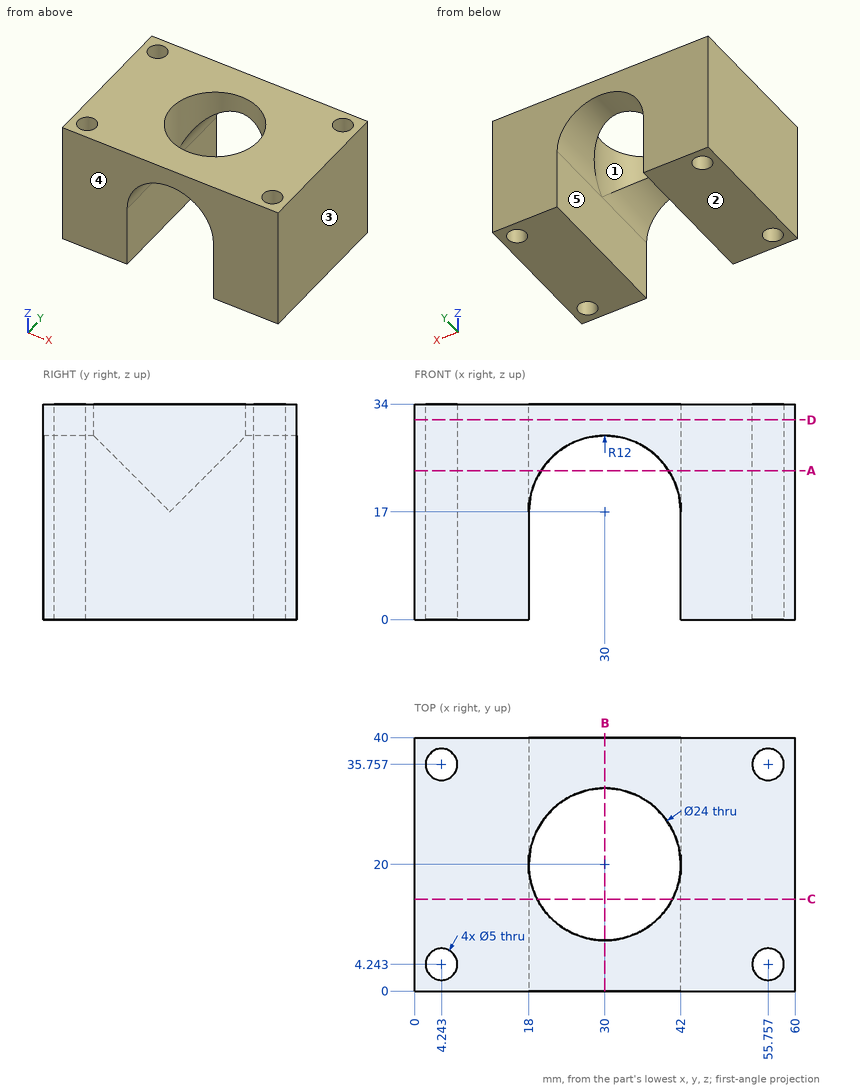
Design review of the part shown in the three views and the two pictorial views. Dimensions are in mm from the part's minimum x, y and z. A direction names the side the tool comes from. Round coordinates to 2 decimals unless told otherwise and drop trailing zeros. Loops run counter-clockwise (first coordinate to the right, second up) from the corner with the lowest first, then second, coordinate; pieces in that order, holes last. Notation, with made-up numbers: M 63,26 L 81,26 A18 ccw 81,35 Z; hole C 51,10.25 d10. An arc over 180 degrees is marked long. Answer as a JSON object with one key per item and string values.
Item 1: Clearance check with a flat-ended pin moving along its axis: P1, Ø8, axis at x = 24.5, y = 22.5, coming from the +Z side. State where the tip first meets the part, or that it passes through.
Answer sheet:
{"P1": "passes through"}
Item 2: We need section D-D on z = 31.5. Give the boundary of the cut face in (x, y), and give its area (3 significant figures).
Answer sheet:
{"outline": "M 0,0 L 60,0 L 60,40 L 0,40 Z; hole C 4.24,4.24 d5; hole C 4.24,35.76 d5; hole C 30,20 d24; hole C 55.76,4.24 d5; hole C 55.76,35.76 d5", "area": "1,870 mm^2"}
Item 3: We need section B-B on x = 30. Give the boundary of the cut face in (y, z), and give its area (3 significant figures).
Answer sheet:
{"outline": "M 0,29 L 8,29 L 8,34 L 0,34 Z; M 32,29 L 40,29 L 40,34 L 32,34 Z", "area": "80.0 mm^2"}
Item 4: We need section C-C on y = 14.5. Give the boundary of the cut face in (x, z) (1 decimal).
Answer sheet:
{"outline": "M 0,0 L 18,0 L 18,17 A12 cw 19.3,22.5 L 19.3,34 L 0,34 Z; M 40.7,22.5 A12 cw 42,17 L 42,0 L 60,0 L 60,34 L 40.7,34 Z"}
Item 5: Machinability: for the marked faces 4 and 5, which of the approach directions +Z, -Z, +X, -X, +Y, -Y give a long, thin tool a straight path to every point of the face, cutting with its end or side? Answer none if there is none.
Answer sheet:
{"face 4": "+Z, -Z, +X, -X, -Y", "face 5": "-Z, +Y, -Y"}
Item 6: We need section A-A on z = 23.5. Give the boundary of the cut face in (x, y), and give its area (3 significant figures).
Answer sheet:
{"outline": "M 0,0 L 19.91,0 L 19.91,13.5 A12 cw 19.91,26.5 L 19.91,40 L 0,40 Z; M 40.09,0 L 60,0 L 60,40 L 40.09,40 L 40.09,26.5 A12 cw 40.09,13.5 Z; hole C 4.24,4.24 d5; hole C 4.24,35.76 d5; hole C 55.76,4.24 d5; hole C 55.76,35.76 d5", "area": "1,480 mm^2"}
Item 7: Wall thickness on L1, parallel to Y at x = 4.5, z = 5.5; L2, parallel to X at y = 19.5, z = 26; L3, parallel to Y at x = 6.5, z = 27 (1 decimal): over which ranges is each line inside the solid? List them lowest first. Write a range as from..to.
Answer sheet:
{"L1": "y = 0..1.76, 6.73..33.27, 38.24..40", "L2": "x = 0..18.01, 41.99..60", "L3": "y = 0..3.2, 5.3..34.7, 36.8..40"}
Item 8: The part is to be moulded in two halves that separate along X. For the marked faces 1, 2 and 3, say which applies: pulls with the +X half, pulls with the -X half, needs draft (parallel to the pull), parting line crosses it, or undercut.
Answer sheet:
{"face 1": "undercut", "face 2": "needs draft", "face 3": "pulls with the +X half"}
